Can you work these out from the drawing? Everything is in mm from the part's minimum corner. Round coordinates to 2 decimals unless told otherwise and drop trailing zeros. Write each loop counter-clockwise with the first axis right and the second up, starting at its lowest first coordinate (ties: lowest second). Pieces come first, ordered by that corner, then holes. Notation, with made-up numbers: (-25, 40.25) -> (-12, 40.25) arc R32 ccw to (-12, 75.25) -> close; hole circle Ø11 at (-11, 89.5). An arc over 180 degrees is marked (long way). Answer as CSV lines item,"result". Start each with the question number.
Q1. Imagine slicing it at C-C on x = 12.5. Please give me the cut outline in (y, z), and give its area (3 significant figures).
Q2. Will these pins go through, and if not, where does the flat tip stop? pin 1 Ø6 at (y, z) = (6.5, 14) entering from +X; pin 2 Ø2 at (x, z) = (7.5, 83.5) entering from -Y; pin 3 Ø5 at (x, z) = (2.5, 51.5) entering from +Y; pin 4 Ø2.5 at (x, y) = (9.5, 6) entering from +Z.
Q3. If we mould it in two halves opening along X, with no side actions, what happens to the marked faces 1 and 2? For each: pulls with the +X half, pulls with the -X half, needs draft (parallel to the pull), parting line crosses it, or undercut.
Q4. If I drill on line 1 (X direction, y = 6.35, z = 5.5); line 2 (Z direction, x = 12, y = 9.25); line 3 (Y direction, x = 17, z = 41), over which ranges is the centre line in solid material (lowest first)? Write a range as [from, to].
Q5. Imagine slicing it at D-D on z = 83. Please give me the cut outline in (x, y).
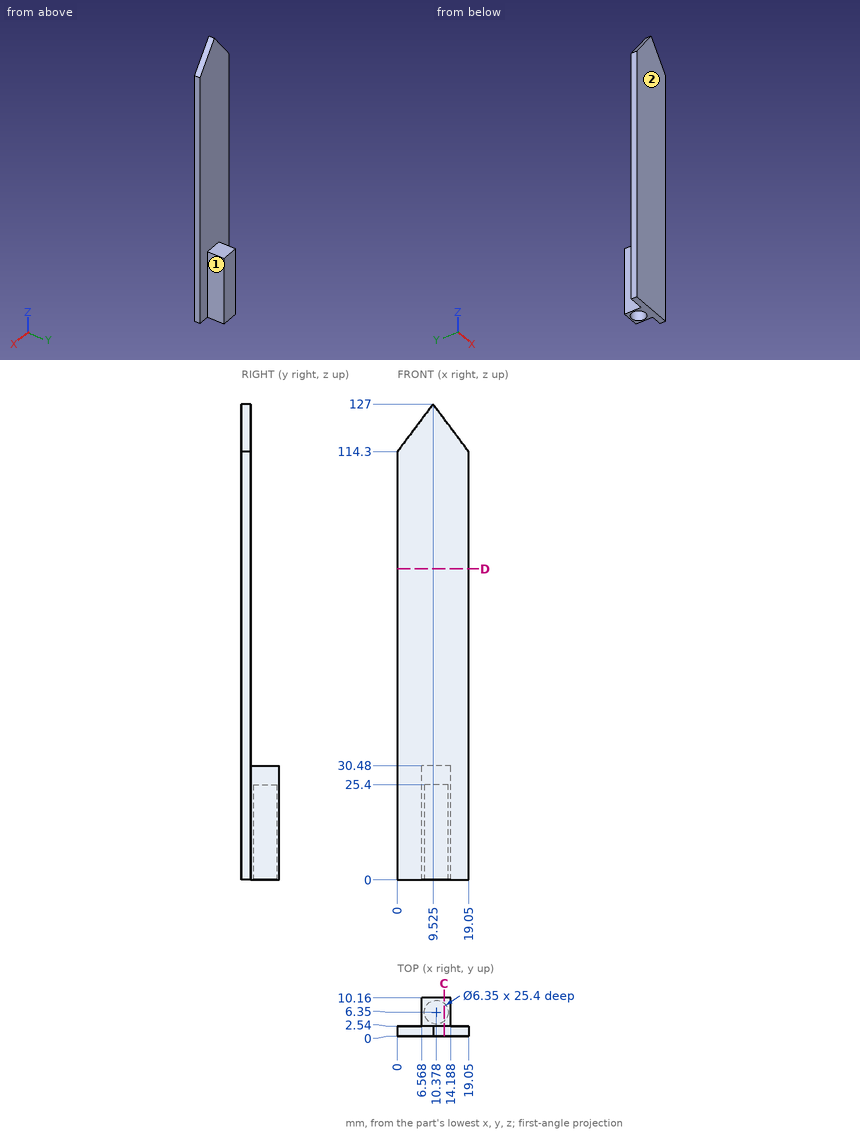
Checks:
1,outline,"(0, 0) -> (3.99, 0) -> (3.99, 25.4) -> (8.71, 25.4) -> (8.71, 0) -> (10.16, 0) -> (10.16, 30.48) -> (2.54, 30.48) -> (2.54, 123.03) -> (0, 123.03) -> close"
1,area,"425 mm^2"
2,pin 1,"x = 14.19"
2,pin 2,"y = 0"
2,pin 3,"y = 2.54"
2,pin 4,"z = 30.48"
3,face 1,"pulls with the +X half"
3,face 2,"needs draft"
4,line 1,"[6.57, 7.2], [13.55, 14.19]"
4,line 2,"[0, 30.48]"
4,line 3,"[0, 2.54]"
5,outline,"(0, 0) -> (19.05, 0) -> (19.05, 2.54) -> (0, 2.54) -> close"
